Drawing for the job (mm, zero at the part's lowest x, y, z). Coordinates: 2 decimals unless noted, no trailing zeros. Order: outer loops, then holes, each group sorted by start corner. A loop starts at its lowest first (then second) coordinate and runs counter-clockwise, first axis right, second up.
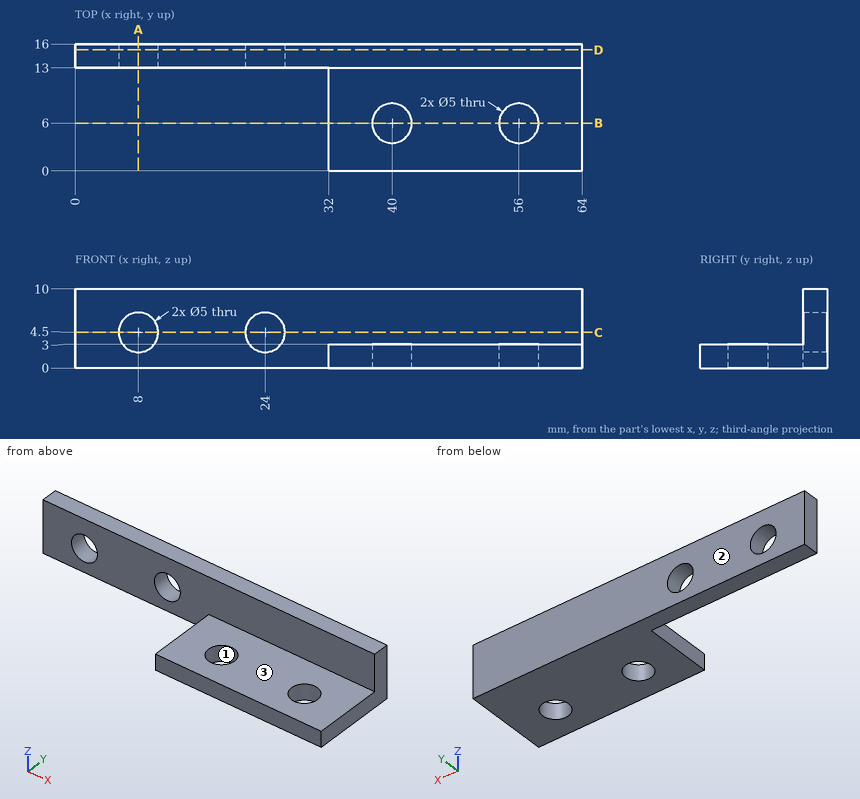
(1) Slice it at A-A, the plane x = 8. Give the cut face in (y, z).
(2) Slice it at D-D, the plane y = 15.25. Give the cut face in (x, z).
(3) Slice it at B-B, the plane y = 6. Give the cut face in (x, z).
(4) Pull direction Y, two halves, no side cores. Call the marked faces 1, 2 and 3: +Y half, -Y half, draft (parallel to the pull), parting line (faces both ways), or undercut.
(5) Slice it at C-C, the plane z = 4.5. Give the cut face in (x, y), then the cut area to 3 significant figures.
(6) Probe line 1 (Z direction, x = 24, y = 14.45); line 2 (X direction, y = 15.25, z = 2.5); line 3 (Z direction, x = 33.5, y = 5.75). List the from-to ranges inside material, lowest first.
(7) Drop flat-ended pins along their axis: pin 1 (5 mm diameter, centred on y = 7.5, z = 1.5, fed in from -X); pin 2 (4 mm diameter, centred on x = 51, y = 4, fed in from +Z); pin 3 (1 mm diameter, centred on x = 29, z = 8.5, fed in from -Y). Give the stop position or say it passes through.
Here are the results:
1. outline: (13, 0) - (16, 0) - (16, 2) - (13, 2) - close; (13, 7) - (16, 7) - (16, 10) - (13, 10) - close
2. outline: (0, 0) - (64, 0) - (64, 10) - (0, 10) - close; hole circle Ø5 at (8, 4.5); hole circle Ø5 at (24, 4.5)
3. outline: (32, 0) - (37.5, 0) - (37.5, 3) - (32, 3) - close; (42.5, 0) - (53.5, 0) - (53.5, 3) - (42.5, 3) - close; (58.5, 0) - (64, 0) - (64, 3) - (58.5, 3) - close
4. face 1: undercut
4. face 2: +Y half
4. face 3: draft
5. outline: (0, 13) - (5.5, 13) - (5.5, 16) - (0, 16) - close; (10.5, 13) - (21.5, 13) - (21.5, 16) - (10.5, 16) - close; (26.5, 13) - (64, 13) - (64, 16) - (26.5, 16) - close
5. area: 162 mm2
6. line 1: z = 0 to 2, 7 to 10
6. line 2: x = 0 to 6.5, 9.5 to 22.5, 25.5 to 64
6. line 3: z = 0 to 3
7. pin 1: stops at x = 32
7. pin 2: stops at z = 3
7. pin 3: stops at y = 13
